```python
from build123d import *

# Parameters (mm, degrees)
SKETCH1_R                                       = 20
SKETCH1_R_2                                     = 2
BOSS_EXTRUDE1_DEPTH                             = 16.25
BOSS_EXTRUDE2_START                             = -3
SKETCH2_R                                       = 20
SKETCH2_R_2                                     = 15
BOSS_EXTRUDE2_DEPTH                             = 3
CSK_FOR_M5_FLAT_HEAD_MACHINE_SCREW1_D           = 4
CSK_FOR_M5_FLAT_HEAD_MACHINE_SCREW1_CSINK_D     = 9
CSK_FOR_M5_FLAT_HEAD_MACHINE_SCREW1_CSINK_ANGLE = 90
CUT_EXTRUDE1_REACH                              = 103.652
SKETCH7_R                                       = 1.65


with BuildPart() as part:
    # Sketch1 → Boss-Extrude1 (new body)
    with BuildSketch(Plane.XY):
        with BuildLine():
            Line((-62, 5), (-9, 5))
            ThreePointArc((-9, 5), (-7.585786438, 4.414213562), (-7, 3))
            Line((-7, 3), (-7, -3))
            ThreePointArc((-7, -3), (-7.585786438, -4.414213562), (-9, -5))
            Line((-9, -5), (-62, -5))
            Line((-62, -5), (-62, -25))
            Line((-62, -25), (62, -25))
            ThreePointArc((62, -25), (87, 0), (62, 25))
            Line((62, 25), (-62, 25))
            Line((-62, 25), (-62, 5))
        make_face()
        with Locations((62, 0)):
            Circle(SKETCH1_R, mode=Mode.SUBTRACT)
        with Locations((-52.5, 17)):
            Circle(SKETCH1_R_2, mode=Mode.SUBTRACT)
        with Locations((-32.5, 17)):
            Circle(SKETCH1_R_2, mode=Mode.SUBTRACT)
        with Locations((-12.5, 17)):
            Circle(SKETCH1_R_2, mode=Mode.SUBTRACT)
        with Locations((-32.5, -17)):
            Circle(SKETCH1_R_2, mode=Mode.SUBTRACT)
        with Locations((-12.5, -17)):
            Circle(SKETCH1_R_2, mode=Mode.SUBTRACT)
        with Locations((-52.5, -17)):
            Circle(SKETCH1_R_2, mode=Mode.SUBTRACT)
    extrude(amount=BOSS_EXTRUDE1_DEPTH)

    # Sketch2 → Boss-Extrude2 (add)
    with BuildSketch(Plane.XY.offset(16.25).offset(BOSS_EXTRUDE2_START)):
        with Locations((62, 0)):
            Circle(SKETCH2_R)
        with Locations((62, 0)):
            Circle(SKETCH2_R_2, mode=Mode.SUBTRACT)
    extrude(amount=BOSS_EXTRUDE2_DEPTH)

    # CSK for M5 Flat Head Machine Screw1 (through all)
    with Locations(Plane.XY.offset(16.25)):
        with Locations((-52.5, 17), (-32.5, 17), (-12.5, 17), (-52.5, -17), (-32.5, -17), (-12.5, -17)):
            CounterSinkHole(CSK_FOR_M5_FLAT_HEAD_MACHINE_SCREW1_D / 2, CSK_FOR_M5_FLAT_HEAD_MACHINE_SCREW1_CSINK_D / 2, counter_sink_angle=CSK_FOR_M5_FLAT_HEAD_MACHINE_SCREW1_CSINK_ANGLE)

    # Sketch7 → Cut-Extrude1 (cut, up to next)
    with BuildSketch(Plane.XZ.offset(25), mode=Mode.PRIVATE) as cut_extrude1_sk1:
        with Locations(Location((-45, 9.25, 0), (0, 0, 270))):
            Circle(SKETCH7_R)
    cut_extrude1_tool1 = extrude(cut_extrude1_sk1.sketch, amount=-CUT_EXTRUDE1_REACH, mode=Mode.PRIVATE) & part.part
    # Sketch7 → Cut-Extrude1 (cut, up to next)
    with BuildSketch(Plane.XZ.offset(25), mode=Mode.PRIVATE) as cut_extrude1_sk2:
        with Locations(Location((-27.943596514, 7.032095554, 0), (0, 0, 270))):
            Circle(SKETCH7_R)
    cut_extrude1_tool2 = extrude(cut_extrude1_sk2.sketch, amount=-CUT_EXTRUDE1_REACH, mode=Mode.PRIVATE) & part.part
    add(cut_extrude1_tool1.solids().sort_by_distance((-45, -25, 9.25))[0], mode=Mode.SUBTRACT)
    add(cut_extrude1_tool2.solids().sort_by_distance((-27.943597, -25, 7.032096))[0], mode=Mode.SUBTRACT)


solid = part.part
```
Input: part model. Units: mm. Frame: model coordinates. A direction names the side the tool comes from. Round coordinates to 2 decimals unless told otherwise and drop trailing zeros. Order: outer loops, then holes, each group sorted by start corner. A loop starts at its lowest first (then second) coordinate and runs counter-clockwise, first axis right, second up. Notation, with made-up numbers: (1.5, 28) - (13.5, 28) arc R20 ccw to (13.5, 49) - close; hole circle Ø1 at (-2, -4.75). An arc over 180 degrees is marked (long way). Answer in a Markdown table with one row per item.
Item 1: Reachability of faces 1 (the cylindrical face through (-29.554, -15.14, 7.39)), 2 (the cylindrical face through (-50.653, 16.234, 6.779)), 3 (the conical face through (-34.46, 16.19, 13.87)), 4 (the flat face through (-36, 5, 8)), 5 (the cylindrical face through (81.076, 6.007, 6.532)) from +Z, -Z, +X, -X, +Y, -Y: full face, straight path, thin tool, end or side. Return the list, or none.
Model answer:
| item | result |
|---|---|
| face 1 | -Y |
| face 2 | +Z, -Z |
| face 3 | +Z |
| face 4 | +Z, -Z, -X |
| face 5 | -Z |
Item 2: Line query: line 1 (Y direction, x = -52.5, z = 10.5); line 2 (Y direction, x = -40.5, z = 13.5); line 3 (X direction, y = -0.5, z = 14.5) (3 decimals). Output: solid intervals per line, ascending.
Model answer:
| item | result |
|---|---|
| line 1 | y = -25 to -19, -15 to -5, 5 to 15, 19 to 25 |
| line 2 | y = -25 to -5, 5 to 25 |
| line 3 | x = -7 to 47.008, 76.992 to 86.995 |
Item 3: Section query A-A (x = -45). Return the cut outline in (y, z).
Model answer:
| item | result |
|---|---|
| outline | (-25, 0) - (-5, 0) - (-5, 7.6) - (-25, 7.6) - close; (-25, 10.9) - (-5, 10.9) - (-5, 16.25) - (-25, 16.25) - close; (5, 0) - (25, 0) - (25, 16.25) - (5, 16.25) - close |
Item 4: Section query D-D (y = -8). Return the cut outline in (x, z).
Model answer:
| item | result |
|---|---|
| outline | (-62, 0) - (43.67, 0) - (43.67, 13.25) - (49.31, 13.25) - (49.31, 16.25) - (-62, 16.25) - close; (74.69, 13.25) - (80.33, 13.25) - (80.33, 0) - (85.69, 0) - (85.69, 16.25) - (74.69, 16.25) - close; hole circle Ø3.3 at (-45, 9.25); hole circle Ø3.3 at (-27.94, 7.03) |
Item 5: Pin query (flat end, axial travel): pin 1 (3.5 mm diameter, centred on x = -12.5, y = 17, fed in from -Z); pin 2 (3 mm diameter, centred on y = 0.5, z = 10.5, fed in from -X); pin 3 (4 mm diameter, centred on x = -27.94, z = 7.03, fed in from -Y); pin 4 (4 mm diameter, centred on y = -2, z = 14.5, fed in from +X). Return the tip coordinate at first contact, or that it passes through.
Model answer:
| item | result |
|---|---|
| pin 1 | passes through |
| pin 2 | stops at x = -7 |
| pin 3 | stops at y = -25 |
| pin 4 | stops at x = 87 |
Item 6: Section query C-C (y = 0). Return the cut outline in (x, z).
Model answer:
| item | result |
|---|---|
| outline | (-7, 0) - (42, 0) - (42, 13.25) - (47, 13.25) - (47, 16.25) - (-7, 16.25) - close; (77, 13.25) - (82, 13.25) - (82, 0) - (87, 0) - (87, 16.25) - (77, 16.25) - close |
Item 7: Mould query, pull axis Z, two halves, no side actions, for faces 6 (the cylindrical face through (-43.364, -15.14, 9.465)), 7 (the flat face through (-62, -15, 8)), 8 (the conical face through (-33.64, -15.21, 13.87)). Classes: released by +Z, released by -Z, zero draft, split by the parting line, or undercut.
Model answer:
| item | result |
|---|---|
| face 6 | undercut |
| face 7 | zero draft |
| face 8 | released by +Z |
Item 8: Section query B-B (z = 1.75). Return the cut outline in (x, y).
Model answer:
| item | result |
|---|---|
| outline | (-62, -25) - (62, -25) arc R25 ccw to (62, 25) - (-62, 25) - (-62, 5) - (-9, 5) arc R2 cw to (-7, 3) - (-7, -3) arc R2 cw to (-9, -5) - (-62, -5) - close; hole circle Ø4 at (-52.5, -17); hole circle Ø4 at (-52.5, 17); hole circle Ø4 at (-32.5, -17); hole circle Ø4 at (-32.5, 17); hole circle Ø4 at (-12.5, -17); hole circle Ø4 at (-12.5, 17); hole circle Ø40 at (62, 0) |
